```python
from build123d import *

# Parameters (mm, degrees)
SKETCH1_W           = 58.42
SKETCH1_H           = 58.42
SKETCH1_R           = 2.55
SKETCH1_R_2         = 5.5
SKETCH1_R_3         = 2.05
BOSS_EXTRUDE1_DEPTH = 6.35
CHAMFER1_SIZE       = 2.48


with BuildPart() as part:
    # Sketch1 → Boss-Extrude1 (new body)
    with BuildSketch(Plane(origin=(0, 0, 0), x_dir=(1, 0, 0), z_dir=(0, 1, 0))):
        with Locations((29.21, 29.21)):
            Rectangle(SKETCH1_W, SKETCH1_H)
        with Locations(Location((5.64, 52.78, 0), (0, 0, 270))):
            Circle(SKETCH1_R, mode=Mode.SUBTRACT)
        with Locations(Location((52.78, 52.78, 0), (0, 0, 270))):
            Circle(SKETCH1_R, mode=Mode.SUBTRACT)
        with Locations(Location((52.78, 5.64, 0), (0, 0, 270))):
            Circle(SKETCH1_R, mode=Mode.SUBTRACT)
        with Locations(Location((5.64, 5.64, 0), (0, 0, 270))):
            Circle(SKETCH1_R, mode=Mode.SUBTRACT)
        with Locations(Location((29.21, 29.21, 0), (0, 0, 270))):
            Circle(SKETCH1_R_2, mode=Mode.SUBTRACT)
        with Locations(Location((13.653650814, 44.766349186, 0), (0, 0, 270))):
            Circle(SKETCH1_R_3, mode=Mode.SUBTRACT)
        with Locations(Location((44.766349186, 44.766349186, 0), (0, 0, 270))):
            Circle(SKETCH1_R_3, mode=Mode.SUBTRACT)
        with Locations(Location((44.766349186, 13.653650814, 0), (0, 0, 270))):
            Circle(SKETCH1_R_3, mode=Mode.SUBTRACT)
        with Locations(Location((13.653650814, 13.653650814, 0), (0, 0, 270))):
            Circle(SKETCH1_R_3, mode=Mode.SUBTRACT)
    extrude(amount=BOSS_EXTRUDE1_DEPTH)

    # Chamfer1
    chamfer1_edges = [part.edges().sort_by_distance(p)[0] for p in [
        (13.653650814, 0, -46.816349186),
        (44.766349186, 0, -46.816349186),
        (44.766349186, 0, -15.703650814),
        (13.653650814, 0, -15.703650814),
    ]]
    chamfer(chamfer1_edges, length=CHAMFER1_SIZE)


solid = part.part
```
Model file for the job. Use its own axes, mm. Give positions to 0.01 mm unless a question says otherwise; leave off trailing zeros. Loops run counter-clockwise (first coordinate to the right, second up) from the corner with the lowest first, then second, coordinate; pieces in that order, holes last. Notation, with made-up numbers: (52.25, 35) -> (103.25, 35) arc R16 cw to (103.25, 59) -> close; hole circle Ø3 at (22, -8.5). An arc over 180 degrees is marked (long way). Write each question's results on one line, items separated by ' | '.
(1) Flat gauge pins, fed straight in: pin 1 Ø6.5 at (x, z) = (5.64, -52.78) entering from +Y; pin 2 Ø3.5 at (x, z) = (44.77, -44.77) entering from +Y. Where does each tip first touch, or does it go through?
Geometry results:
pin 1: stops at y = 6.35 | pin 2: passes through
(2) Cut at B-B on z = -52.78. List the corners of the cut face in (x, y).
Geometry results:
outline: (0, 0) -> (3.09, 0) -> (3.09, 6.35) -> (0, 6.35) -> close; (8.19, 0) -> (50.23, 0) -> (50.23, 6.35) -> (8.19, 6.35) -> close; (55.33, 0) -> (58.42, 0) -> (58.42, 6.35) -> (55.33, 6.35) -> close
(3) Cut at C-C on x = 52.78. List the corners of the cut face in (y, z), and give its area (3 significant figures).
Geometry results:
outline: (0, -58.42) -> (6.35, -58.42) -> (6.35, -55.33) -> (0, -55.33) -> close; (0, -50.23) -> (6.35, -50.23) -> (6.35, -8.19) -> (0, -8.19) -> close; (0, -3.09) -> (6.35, -3.09) -> (6.35, 0) -> (0, 0) -> close | area: 306 mm²
(4) Cut at A-A on x = 29.21. List the corners of the cut face in (y, z), and give its area (3 significant figures).
Geometry results:
outline: (0, -58.42) -> (6.35, -58.42) -> (6.35, -34.71) -> (0, -34.71) -> close; (0, -23.71) -> (6.35, -23.71) -> (6.35, 0) -> (0, 0) -> close | area: 301 mm²
(5) Pull direction X, two halves, no side cores. Call faces 1 (the conical face through (15.144, 2.325, -15.279)), 2 (the flat face through (29, 0, -36)), 3 (the flat face through (58.42, 3, -29)): released by +X, released by -X, zero draft, split by the parting line, or undercut.
Geometry results:
face 1: undercut | face 2: zero draft | face 3: released by +X
(6) Cut at D-D on y = 3.25. Give the number of separate pieces and of enclosed holes in the cut face, and give its area (3 significant figures).
Geometry results:
separate pieces: 1 | enclosed holes: 9 | area: 3,180 mm²
(7) Probe line 1 along X through (y, z) = (4.25, -52.78); line 2 along Z through (x, y) = (29.5, 3.25); line 3 along X through (y, z) = (4.5, -46). List the from-to ranges inside material, lowest first.
Geometry results:
line 1: x = 0 to 3.09, 8.19 to 50.23, 55.33 to 58.42 | line 2: z = -58.42 to -34.7, -23.72 to 0 | line 3: x = 0 to 12.02, 15.29 to 43.13, 46.4 to 58.42
